Input: part model. Units: mm. Frame: model coordinates. A direction names the side the tool comes from. Round coordinates to 2 decimals unless told otherwise and drop trailing zeros. Loops run counter-clockwise (first coordinate to the right, second up) from the corner with the lowest first, then second, coordinate; pieces in that order, holes last. Notation, with made-up numbers: M 33,36.5 L 41,36.5 A27 cw 41,58.5 Z; hole C 35.5,39 d1. An arc over 180 degrees is marked long. Return JSON: item names as keys, results as strings. Group by question number.
1) Mould query, pull axis Z, two halves, no side actions, for faces 1 (the face through (-3, 1, -43)), 2 (the face through (-29, -12, 52)), 3 (the face through (-1, -40, 9)), 4 (the face through (-62.047, -37.868, -50.479)). Classes: +Z half, -Z half, draft (parallel to the pull), parting line (faces both ways), or undercut.
2) Access query for faces 5 (the face through (-51, -10, -50)), 6 (the face through (-62.047, -37.868, 50.521)), 7 (the face through (-30, -22, -49)). Directions: +Z, -Z, +X, -X, +Y, -Y. A direction counts if a zero-diameter tool reaches every point of the face in a straight line with its end or side. Return the directions, or none.
3) Section A-A (z = 0). Output: boundary loops of the cut face in (x, y).
4) Section B-B (x = -14.05). Output: boundary loops of the cut face in (y, z).
5) Section C-C (x = -29). Output: boundary loops of the cut face in (y, z).
6) Material intervals for line 1 (Z direction, x = -10.5, y = -7); line 2 (X direction, y = 41.5, z = -13), sorted ascending. Write a range as from..to.
7) Contact query for flat-ended pins moving along their axis: P1, Ø7, axis at y = 35.36, z = 35.36, coming from the -X side; P2, Ø3.5, axis at x = -46, z = 51, coming from the +Y side. Output: stop coordinate, or through.
8) Section D-D (y = 8.5). Output: boundary loops of the cut face in (x, z), plus the area to 3 significant figures.
from build123d import *

# Parameters (mm, degrees)
SKETCH_1_W                         = 98
SKETCH_1_H                         = 100
SKETCH_1_R                         = 41
SKETCH_1_R_2                       = 3
SM_BASE_FLANGE_1_DEPTH             = 3
SM_EDGE_FLANGE_1_STRIP_W           = 12.2
SM_EDGE_FLANGE_1_STRIP_H           = 3
SM_EDGE_FLANGE_1_STRIP_CUT_DEPTH   = 100
SM_EDGE_FLANGE_1_STRIP_2_W         = 12.2
SM_EDGE_FLANGE_1_STRIP_2_H         = 3
SM_EDGE_FLANGE_1_STRIP_CUT_2_DEPTH = 100
SM_EDGE_FLANGE_1_DEPTH             = 100
SM_EDGE_FLANGE_1_BEND_DEPTH        = 100
SKETCH_8_R                         = 3
CUT_EXTRUDE_1_DEPTH                = 135.96666255
FILLET_1_R                         = 8


# Sheet-metal steps are written as plain solids
with BuildPart() as part:
    # Sketch 1 → 基体-法兰1 (new body)
    with BuildSketch(Plane(origin=(0, 0, 0), x_dir=(0, 0, -1), z_dir=(1, 0, 0))):
        Rectangle(SKETCH_1_W, SKETCH_1_H)
        Circle(SKETCH_1_R, mode=Mode.SUBTRACT)
        with Locations((-35.355339059, 35.355339059)):
            Circle(SKETCH_1_R_2, mode=Mode.SUBTRACT)
        with Locations((35.355339059, 35.355339059)):
            Circle(SKETCH_1_R_2, mode=Mode.SUBTRACT)
        with Locations((35.355339059, -35.355339059)):
            Circle(SKETCH_1_R_2, mode=Mode.SUBTRACT)
        with Locations((-35.355339059, -35.355339059)):
            Circle(SKETCH_1_R_2, mode=Mode.SUBTRACT)
    extrude(amount=-SM_BASE_FLANGE_1_DEPTH)

    # 边线-法兰1 strip (across the edge) → 边线-法兰1 strip cut (cut)
    with BuildSketch(Plane(origin=(-3, -50, 49), x_dir=(0, 0, -1), z_dir=(0, 1, 0))):
        with Locations((-6, -1.5)):
            Rectangle(SM_EDGE_FLANGE_1_STRIP_W, SM_EDGE_FLANGE_1_STRIP_H)
    extrude(amount=SM_EDGE_FLANGE_1_STRIP_CUT_DEPTH, mode=Mode.SUBTRACT)

    # 边线-法兰1 strip 2 (across the edge) → 边线-法兰1 strip cut 2 (cut)
    with BuildSketch(Plane(origin=(-3, 50, -49), x_dir=(0, 0, 1), z_dir=(0, -1, 0))):
        with Locations((-6, -1.5)):
            Rectangle(SM_EDGE_FLANGE_1_STRIP_2_W, SM_EDGE_FLANGE_1_STRIP_2_H)
    extrude(amount=SM_EDGE_FLANGE_1_STRIP_CUT_2_DEPTH, mode=Mode.SUBTRACT)

    # 边线-法兰1 section (across the edge) → 边线-法兰1 (add)
    with BuildSketch(Plane(origin=(-3, -50, 49), x_dir=(0, 0, -1), z_dir=(0, 1, 0))):
        with BuildLine():
            Line((-3, 0.1), (-3, 67))
            Line((-3, 67), (0, 67))
            Line((0, 67), (0, 0.1))
            ThreePointArc((0, 0.1), (0.029289322, 0.029289322), (0.1, 0))
            Line((0.1, 0), (0.1, -3))
            ThreePointArc((0.1, -3), (-2.092031022, -2.092031022), (-3, 0.1))
        make_face()
    extrude(amount=SM_EDGE_FLANGE_1_DEPTH)

    # 边线-法兰1 section 2 (across the edge) → 边线-法兰1 bend (add)
    with BuildSketch(Plane(origin=(-3, 50, -49), x_dir=(0, 0, 1), z_dir=(0, -1, 0))):
        with BuildLine():
            Line((-3, 0.1), (-3, 67))
            Line((-3, 67), (0, 67))
            Line((0, 67), (0, 0.1))
            ThreePointArc((0, 0.1), (0.029289322, 0.029289322), (0.1, 0))
            Line((0.1, 0), (0.1, -3))
            ThreePointArc((0.1, -3), (-2.092031022, -2.092031022), (-3, 0.1))
        make_face()
    extrude(amount=SM_EDGE_FLANGE_1_BEND_DEPTH)

    # 草图8 → 切除-拉伸1 (cut, through all)
    with BuildSketch(Plane.XY.offset(52)):
        with Locations((-14.05, -38)):
            Circle(SKETCH_8_R)
        with Locations((-59.05, -38)):
            Circle(SKETCH_8_R)
        Polygon((-10, 50), (-70, 50), (-70, -10), (-35, -10), align=None)
    extrude(amount=-CUT_EXTRUDE_1_DEPTH, mode=Mode.SUBTRACT)

    # 圆角1
    fillet_1_edges = [part.edges().sort_by_distance(p)[0] for p in [
        (-10, 50, 50.5),
        (-70, -10, 50.5),
        (-35, -10, 50.5),
        (-10, 50, -50.5),
        (-35, -10, -50.5),
        (-70, -10, -50.5),
        (-70, -50, 50.5),
        (-70, -50, -50.5),
    ]]
    fillet(fillet_1_edges, radius=FILLET_1_R)


solid = part.part
Returned:
{
 "1": {"face 1": "undercut", "face 2": "+Z half", "face 3": "undercut", "face 4": "draft"},
 "2": {"face 5": "+Z, -Z, -X, +Y", "face 6": "+Z, -Z", "face 7": "-X, +Y, -Y"},
 "3": {"outline": "M -3,-50 L 0,-50 L 0,-41 L -3,-41 Z; M -3,41 L 0,41 L 0,50 L -3,50 Z"},
 "4": {"outline": "M -50,-52 L -41,-52 L -41,-49 L -50,-49 Z; M -50,49 L -41,49 L -41,52 L -50,52 Z; M -35,-52 L 40.28,-52 L 40.28,-49 L -35,-49 Z; M -35,49 L 40.28,49 L 40.28,52 L -35,52 Z"},
 "5": {"outline": "M -50,-52 L 4.4,-52 L 4.4,-49 L -50,-49 Z; M -50,49 L 4.4,49 L 4.4,52 L -50,52 Z"},
 "6": {"line 1": "z = -52..-49, 49..52", "line 2": "x = -3..0"},
 "7": {"P1": "stops at x = -3", "P2": "stops at y = -10"},
 "8": {"outline": "M -27.29,-52 L -3.1,-52 A3.1 ccw 0,-48.9 L 0,-40.11 L -3,-40.11 L -3,-48.9 A0.1 cw -3.1,-49 L -27.29,-49 Z; M -27.29,49 L -3.1,49 A0.1 cw -3,48.9 L -3,40.11 L 0,40.11 L 0,48.9 A3.1 ccw -3.1,52 L -27.29,52 Z", "area": "213 mm^2"}
}
